Design review of the part shown in the three views and the two pictorial views. Dimensions are in mm from the part's minimum x, y and z. A direction names the side the tool comes from. Round coordinates to 2 decimals unless told otherwise and drop trailing zeros. Loops run counter-clockwise (first coordinate to the right, second up) from the corner with the lowest first, then second, coordinate; pieces in that order, holes last.
1. Tool access review of the marked faces 4 and 5: name each direction out of +Z, -Z, +X, -X, +Y, -Y from which nothing blocks a thin tool from reaching the whole face with its end or side.
2. Consider section A-A on z = 112. State the section outline as (x, y) points, then the cut area to 3 significant figures.
3. To check wall thickness, follow line 1 along X through (y, z) = (132, 60); line 2 along Z through (x, y) = (7, 138); line 3 along Y through (x, z) = (58, 140) (1 decimal). State the ranges of each line that lie inside material, in increasing order.
4. Clearance check with flat-ended pins moving along their axes: pin 1 Ø1.5 at (y, z) = (127, 60.5) entering from -X; pin 2 Ø2 at (x, z) = (61.5, 33) entering from -Y; pin 3 Ø10 at (y, z) = (103, 67.5) entering from +X; pin 4 Ø15 at (x, y) = (36.5, 114) entering from +Z. State where each tip first meets the part, or that it passes through.
5. Draft analysis for pull direction Y (two halves, no side actions). For the marked faces 1, 2 and 3, state which applies: released by +Y, released by -Y, zero draft, split by the parting line, or undercut.
6. Consider section B-B on y = 48.5. State the section outline as (x, z) points.
7. Consider section D-D on z = 30. State the section outline as (x, y) points.
8. Consider section C-C on x = 57. State the section outline as (y, z) points (1 decimal).
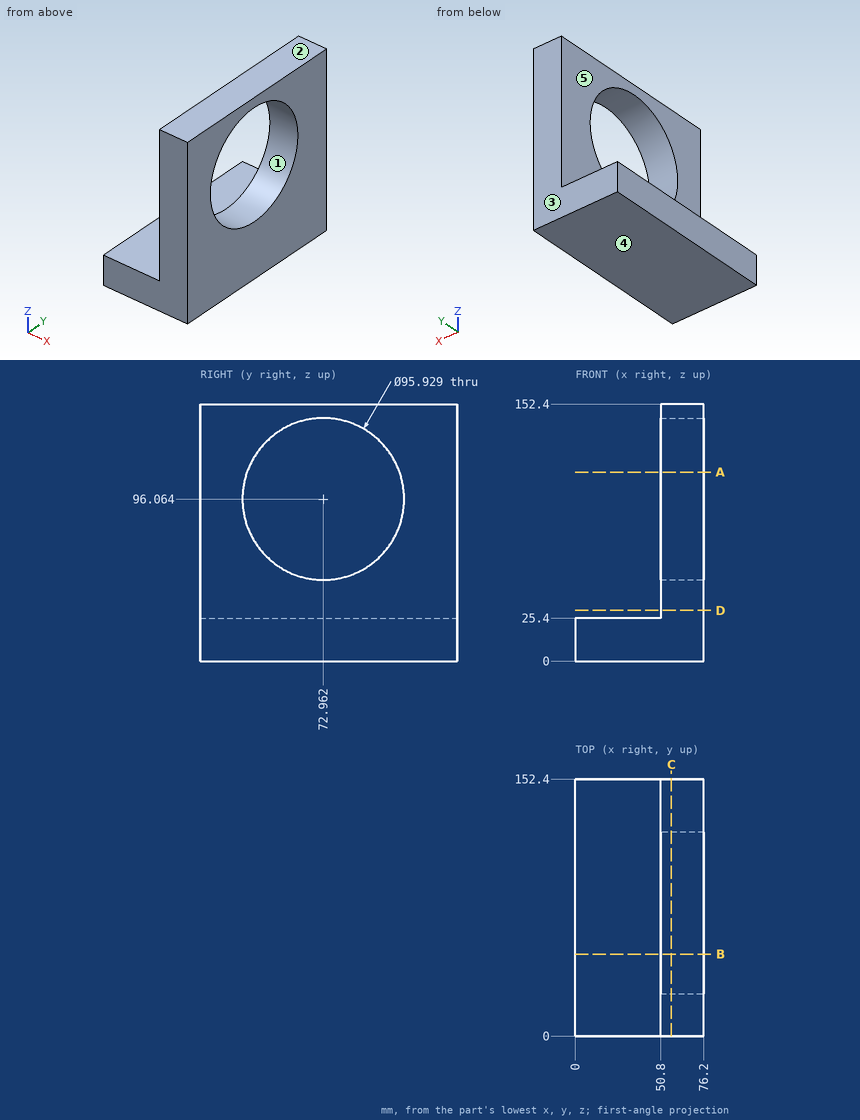
Resolved:
1. face 4: -Z, +X, -X, +Y, -Y
1. face 5: +Z, -X, +Y, -Y
2. outline: (50.8, 0) - (76.2, 0) - (76.2, 27.72) - (50.8, 27.72) - close; (50.8, 118.2) - (76.2, 118.2) - (76.2, 152.4) - (50.8, 152.4) - close
2. area: 1,570 mm2
3. line 1: x = 50.8 to 76.2
3. line 2: z = 0 to 25.4
3. line 3: y = 0 to 53.7, 92.2 to 152.4
4. pin 1: stops at x = 50.8
4. pin 2: stops at y = 0
4. pin 3: passes through
4. pin 4: stops at z = 25.4
5. face 1: undercut
5. face 2: zero draft
5. face 3: released by +Y
6. outline: (0, 0) - (76.2, 0) - (76.2, 54.81) - (50.8, 54.81) - (50.8, 25.4) - (0, 25.4) - close; (50.8, 137.32) - (76.2, 137.32) - (76.2, 152.4) - (50.8, 152.4) - close
7. outline: (50.8, 0) - (76.2, 0) - (76.2, 152.4) - (50.8, 152.4) - close
8. outline: (0, 0) - (152.4, 0) - (152.4, 152.4) - (0, 152.4) - close; hole circle Ø95.9 at (73, 96.1)
